from build123d import *

# Parameters (mm, degrees)
SKETCH1_R           = 2.75
SKETCH1_R_2         = 15
SKETCH1_R_3         = 5
BOSS_EXTRUDE3_DEPTH = 3


with BuildPart() as part:
    # Sketch1 → Boss-Extrude3 (new body)
    with BuildSketch(Plane(origin=(0, 0, 0), x_dir=(1, 0, 0), z_dir=(0, 1, 0))):
        with BuildLine():
            Line((-17.506658739, 0), (-18.165165803, 0))
            ThreePointArc((-18.165165803, 0), (-21.149463035, -1.424316358), (-22.376192782, -4.495121005))
            Line((-22.376192782, -4.495121005), (-14.295317192, -200.74104694))
            ThreePointArc((-14.295317192, -200.74104694), (-15.017989675, -204.775435104), (-17.298404685, -208.181055571))
            ThreePointArc((-17.298404685, -208.181055571), (0, -201.226886238), (17.298404685, -208.181055571))
            ThreePointArc((17.298404685, -208.181055571), (15.017989675, -204.775435104), (14.295317192, -200.74104694))
            Line((14.295317192, -200.74104694), (22.376192782, -4.495121005))
            ThreePointArc((22.376192782, -4.495121005), (21.149463035, -1.424316358), (18.165165803, 0))
            Line((18.165165803, 0), (17.506658739, 0))
            Line((17.506658739, 0), (-17.506658739, 0))
        make_face()
        with Locations((-11.757886925, -10.70503214)):
            Circle(SKETCH1_R, mode=Mode.SUBTRACT)
        with Locations((0.008138346, -11.218747897)):
            Circle(SKETCH1_R, mode=Mode.SUBTRACT)
        with Locations((11.774163618, -10.70503214)):
            Circle(SKETCH1_R, mode=Mode.SUBTRACT)
        with BuildLine():
            ThreePointArc((17.298404685, -208.181055571), (0, -201.226886238), (-17.298404685, -208.181055571))
            ThreePointArc((-17.298404685, -208.181055571), (-17.349081254, -208.230277568), (-17.400104292, -208.279140328))
            ThreePointArc((-17.400104292, -208.279140328), (-9.739921707, -249.234548423), (24.991861654, -226.218747892))
            ThreePointArc((24.991861654, -226.218747892), (23.015800531, -216.478826185), (17.400104292, -208.279140328))
            ThreePointArc((17.400104292, -208.279140328), (17.349081254, -208.230277568), (17.298404685, -208.181055571))
        make_face()
        with Locations((0, -226.218747892)):
            Circle(SKETCH1_R_2, mode=Mode.SUBTRACT)
        with Locations((0, -226.218747892)):
            Circle(SKETCH1_R_2)
        with Locations((0, -226.218747892)):
            Circle(SKETCH1_R_3, mode=Mode.SUBTRACT)
        with Locations((0, -226.218747892)):
            Circle(SKETCH1_R_3)
    extrude(amount=BOSS_EXTRUDE3_DEPTH)


solid = part.part
For this review, take the finished solid that the model builds, in its own axes (mm). A direction names the side the tool comes from. Coordinates: 2 decimals unless noted, no trailing zeros. Loops run counter-clockwise (first coordinate to the right, second up) from the corner with the lowest first, then second, coordinate; pieces in that order, holes last. Notation, with made-up numbers: (87.25, -29) - (113.25, -29) arc R28 cw to (113.25, 3) - close; hole circle Ø7 at (26.25, -10). An arc over 180 degrees is marked (long way). Return JSON: item names as keys, results as strings.
Item 1: Take a section at B-B (y = 0.65). Give the boundary of the cut face in (x, z).
Determined:
{"outline": "(-22.38, 4.5) arc R4.54 ccw to (-18.17, 0) - (18.17, 0) arc R4.54 ccw to (22.38, 4.5) - (14.3, 200.74) arc R10 cw to (17.3, 208.18) arc R10 cw to (17.4, 208.28) arc R24.99 ccw (long way) to (-17.4, 208.28) arc R10 cw to (-17.3, 208.18) arc R10 cw to (-14.3, 200.74) - close; hole circle Ø5.5 at (-11.76, 10.71); hole circle Ø5.5 at (0.01, 11.22); hole circle Ø5.5 at (11.77, 10.71)"}
Item 2: Take a section at D-D (z = 150). Give the boundary of the cut face in (x, y), then the cut area to 3 significant figures.
Determined:
{"outline": "(-16.38, 0) - (16.38, 0) - (16.38, 3) - (-16.38, 3) - close", "area": "98.3 mm2"}
Item 3: Take a section at C-C (z = 102.5). Give the boundary of the cut face in (x, y).
Determined:
{"outline": "(-18.34, 0) - (18.34, 0) - (18.34, 3) - (-18.34, 3) - close"}
Item 4: For line 1 (Z direction, x = -9.5, y = 2.45); line 2 (Z direction, x = 0, y = 0.3); line 3 (Z direction, x = -5, y = 0.4), list the stretches that pass through material, from the lowest coordinate up.
Determined:
{"line 1": "z = 0 to 9.14, 12.27 to 249.33", "line 2": "z = 0 to 8.47, 13.97 to 251.21", "line 3": "z = 0 to 250.71"}
Item 5: For faces 1 (the flat face through (-18.392, 1.479, 101.244)), 2 (the cylindrical face through (-21.117, 1.479, 1.39)), list the 3-axis set-ups (+Z, -Z, +X, -X, +Y, -Y) from which the entire face can be reached by the end or side of a thin tool; tool diameter is ignored.
Determined:
{"face 1": "-X, +Y, -Y", "face 2": "-Z, -X, +Y, -Y"}
Item 6: Take a section at A-A (x = 0). Give the boundary of the cut face in (y, z).
Determined:
{"outline": "(0, 0) - (3, 0) - (3, 8.47) - (0, 8.47) - close; (0, 13.97) - (3, 13.97) - (3, 251.21) - (0, 251.21) - close"}
Item 7: Mouldability with a two-part tool opening along X and no side actions: class faces 3 (the cylindrical face through (-12.12, 1.48, 7.98)), 4 (the flat face through (18.28, 1.48, 103.99)), 5 (the flat face through (0, 3, 124)) as pulls with the +X half, pulls with the -X half, needs draft (parallel to the pull), parting line crosses it, or undercut.
Determined:
{"face 3": "undercut", "face 4": "pulls with the +X half", "face 5": "needs draft"}
Item 8: Insertion check: pin 1 (8 mm diameter, centred on x = -2.5, z = 147, fed in from -Y); pin 2 (1.5 mm diameter, centred on y = 2, z = 92.5, fed in from +X); pin 3 (1 mm diameter, centred on x = 19, y = 1, fed in from -Z). Each pin has a flat end and moves straight along its axis. Give the tip position at first contact, or say it passes through.
Determined:
{"pin 1": "stops at y = 0", "pin 2": "stops at x = 18.78", "pin 3": "stops at z = 0.04"}
